```python
from build123d import *

# Parameters (mm, degrees)
SKETCH155_R     = 1.55
SKETCH155_R_2   = 2.05
SKETCH155_R_3   = 1.05
PAD061_DEPTH    = 4
POCKET077_DEPTH = 4.001
POCKET078_DEPTH = 4.001
FILLET005_R     = 0.8


with BuildPart() as part:
    # Sketch155 → Pad061 (new body)
    with BuildSketch(Plane.XY):
        with BuildLine():
            Line((-22, 28), (-45, 28))
            ThreePointArc((-45, 28), (-48.535534, 26.535534), (-50, 23))
            Line((-50, 23), (-50, 13.15))
            ThreePointArc((-51.5, 11.65), (-50.43934, 12.08934), (-50, 13.15))
            Line((-51.5, 11.65), (-54.8, 11.65))
            ThreePointArc((-54.8, 11.65), (-55.86066, 11.21066), (-56.3, 10.15))
            Line((-56.3, 10.15), (-56.3, -14.47))
            ThreePointArc((-56.3, -14.47), (-55.86066, -15.53066), (-54.8, -15.97))
            Line((-51.5, -15.97), (-54.8, -15.97))
            ThreePointArc((-50, -17.47), (-50.43934, -16.40934), (-51.5, -15.97))
            Line((-50, -17.47), (-50, -30))
            ThreePointArc((-50, -30), (-48.535534, -33.535534), (-45, -35))
            Line((-45, -35), (-22, -35))
            ThreePointArc((-22, -35), (-18.751973, -34.644122), (-15.658065, -33.593376))
            Line((-15.658065, -33.593376), (2.229785, -25.247871))
            ThreePointArc((2.229785, -25.247871), (3.702054, -23.956343), (4.25, -22.076084))
            Line((4.25, 22.076084), (4.25, -22.076084))
            ThreePointArc((4.25, 22.076084), (3.365413, 24.401942), (1.158791, 25.552129))
            Line((-17.328103, 27.72623), (1.158791, 25.552129))
            ThreePointArc((-17.328103, 27.72623), (-19.660044, 27.931499), (-22, 28))
        make_face()
        with Locations((-3, 21.75)):
            Circle(SKETCH155_R, mode=Mode.SUBTRACT)
        with Locations((-3, -21.75)):
            Circle(SKETCH155_R, mode=Mode.SUBTRACT)
        with Locations((-3, 0)):
            Circle(SKETCH155_R_2, mode=Mode.SUBTRACT)
        with Locations((-42.5, -30.7)):
            Circle(SKETCH155_R_2, mode=Mode.SUBTRACT)
        with Locations((-27.5, -30.7)):
            Circle(SKETCH155_R_2, mode=Mode.SUBTRACT)
        with Locations((-42.5, 23.3)):
            Circle(SKETCH155_R_2, mode=Mode.SUBTRACT)
        with Locations((-27.5, 23.3)):
            Circle(SKETCH155_R_2, mode=Mode.SUBTRACT)
        with Locations((-52.65, 8)):
            Circle(SKETCH155_R_3, mode=Mode.SUBTRACT)
        with Locations((-52.65, -12.32)):
            Circle(SKETCH155_R_3, mode=Mode.SUBTRACT)
    extrude(amount=PAD061_DEPTH)

    # Sketch156 (on Face31 of Pad061) → Pocket077 (cut, through all)
    with BuildSketch(Plane.XY.offset(4)):
        with BuildLine():
            Line((-42.5, -26.5), (-30.5, -26.5))
            ThreePointArc((-30.5, -26.5), (-29.085786, -25.914214), (-28.5, -24.5))
            Line((-28.5, -24.5), (-28.5, -15))
            ThreePointArc((-28.5, -15), (-29.085786, -13.585786), (-30.5, -13))
            Line((-30.5, -13), (-42.5, -13))
            ThreePointArc((-42.5, -13), (-43.914214, -13.585786), (-44.5, -15))
            Line((-44.5, -15), (-44.5, -24.5))
            ThreePointArc((-44.5, -24.5), (-43.914214, -25.914214), (-42.5, -26.5))
        make_face()
        with BuildLine():
            Line((-41, -7.5), (-32, -7.5))
            ThreePointArc((-32, -7.5), (-29.87868, -6.62132), (-29, -4.5))
            Line((-29, -4.5), (-29, 4.5))
            ThreePointArc((-29, 4.5), (-29.87868, 6.62132), (-32, 7.5))
            Line((-32, 7.5), (-41, 7.5))
            ThreePointArc((-41, 7.5), (-43.12132, 6.62132), (-44, 4.5))
            Line((-44, 4.5), (-44, -4.5))
            ThreePointArc((-44, -4.5), (-43.12132, -6.62132), (-41, -7.5))
        make_face()
        with BuildLine():
            Line((-40.5, 13), (-32.5, 13))
            ThreePointArc((-32.5, 13), (-31.085786, 13.585786), (-30.5, 15))
            Line((-30.5, 15), (-30.5, 18.5))
            ThreePointArc((-30.5, 18.5), (-31.085786, 19.914214), (-32.5, 20.5))
            Line((-32.5, 20.5), (-40.5, 20.5))
            ThreePointArc((-40.5, 20.5), (-41.914214, 19.914214), (-42.5, 18.5))
            Line((-42.5, 18.5), (-42.5, 15))
            ThreePointArc((-42.5, 15), (-41.914214, 13.585786), (-40.5, 13))
        make_face()
    extrude(amount=-POCKET077_DEPTH, mode=Mode.SUBTRACT)

    # Sketch157 (on Face5 of Pocket077) → Pocket078 (cut, through all)
    with BuildSketch(Plane.XY.offset(4)):
        with BuildLine():
            ThreePointArc((-7.582576, -2), (-4.119662, -4.873023), (0.25, -3.799671))
            Line((0.25, -3.799671), (0.25, -19.418155))
            ThreePointArc((0.25, -19.418155), (-1.755149, -17.948639), (-4.241129, -17.947422))
            Line((-4.241129, -17.947422), (-22, -2))
            Line((-22, -2), (-7.582576, -2))
        make_face()
        with BuildLine():
            ThreePointArc((-6.93352, 22.476238), (-6.999674, 21.698928), (-6.913694, 20.92356))
            Line((-22, 7.376095), (-6.913694, 20.92356))
            Line((-22, 24), (-22, 7.376095))
            ThreePointArc((-17.795293, 23.753607), (-19.89404, 23.938349), (-22, 24))
            Line((-6.93352, 22.476238), (-17.795293, 23.753607))
        make_face()
        with BuildLine():
            Line((0.25, 19.418155), (0.25, 3.799671))
            ThreePointArc((0.25, 3.799671), (-4.119662, 4.873023), (-7.582576, 2))
            Line((-22, 2), (-7.582576, 2))
            Line((-4.241129, 17.947422), (-22, 2))
            ThreePointArc((-4.241129, 17.947422), (-1.755149, 17.948639), (0.25, 19.418155))
        make_face()
        with BuildLine():
            Line((-17.349248, -29.968476), (-5.818135, -24.588681))
            ThreePointArc((-6.913694, -20.92356), (-6.832448, -22.895575), (-5.818135, -24.588681))
            Line((-6.913694, -20.92356), (-22, -7.376095))
            Line((-22, -7.376095), (-22, -31))
            ThreePointArc((-22, -31), (-19.618113, -30.739023), (-17.349248, -29.968476))
        make_face()
    extrude(amount=-POCKET078_DEPTH, mode=Mode.SUBTRACT)

    # Fillet005
    fillet005_edges = [part.edges().sort_by_distance(p)[0] for p in [
        (-22, -7.376095, 2),
        (-22, -2, 2),
        (-6.913694, -20.92356, 2),
        (-5.818135, -24.588681, 2),
        (-22, -31, 2),
        (-22, 2, 2),
        (-4.241129, 17.947422, 2),
        (0.25, 19.418155, 2),
        (-7.582576, 2, 2),
        (0.25, 3.799671, 2),
        (-22, 7.376095, 2),
        (-22, 24, 2),
        (-6.93352, 22.476238, 2),
        (-6.913694, 20.92356, 2),
        (0.25, -3.799671, 2),
        (-7.582576, -2, 2),
        (-4.241129, -17.947422, 2),
        (0.25, -19.418155, 2),
    ]]
    fillet(fillet005_edges, radius=FILLET005_R)


with BuildPart() as part_1:
    # Body023 placement: moved
    add(part.part.moved(Location((0, 0, 8.1))))


solid = part_1.part
```
Model file for the job. Use its own axes, mm. A direction names the side the tool comes from. Round coordinates to 2 decimals unless told otherwise and drop trailing zeros. Loops run counter-clockwise (first coordinate to the right, second up) from the corner with the lowest first, then second, coordinate; pieces in that order, holes last. Notation, with made-up numbers: M 47.5,-11.5 L 80.5,-11.5 A20 cw 80.5,-3.5 Z; hole C -24,13.25 d2. An arc over 180 degrees is marked long. Put each result on its own line as item: value. Start each with the question number.
Item 1: Cut at B-B (y = -6.5). List the corners of the cut face in (x, z), then the cut area to 3 significant figures.
Item 2: Drill centre lines: line 1 along Y through (x, z) = (-27.5, 9.75); line 2 along Y through (x, z) = (-52.65, 10.7); line 3 along Y through (x, z) = (-41, 8.7). Where is each one in solid material? Low to high.
Item 3: 3-axis set-ups, long thin cutter, end or side, ignore diameter. For faces 1 (the face through (-50, 18, 10)), 2 (the face through (-31.07, 19.9, 10.13)), 3 (the face through (-56.3, -2, 10)): which of +Z, -Z, +X, -X, +Y, -Y reach the whole face in a straight line?
Item 4: Cut at C-C (x = -3). List the corners of the cut face in (y, z), then the cut area to 3 significant figures.
Item 5: Mould opens along X. For faces 4 (the face through (-48, 27, 10)), 5 (the face through (-43.9, -13.57, 10.13)), 6 (the face through (-2.38, 17.8, 10.13)), 7 (the face through (-53, 11.65, 10)) say: released by +X, released by -X, zero draft, split by the parting line, or undercut.
Item 6: Cut at D-D (x = -12). List the corners of the cut face in (y, z), then the cut area to 3 significant figures.
Item 7: Drop flat-ended pins along their axis: P1, Ø1.5, axis at y = -24.5, z = 10.5, coming from the -X side; P2, Ø1.2, axis at y = 12, z = 10.5, coming from the -X side; P3, Ø1, axis at x = -53.5, z = 10.5, coming from the +Y side. Give the stop position or say it passes through.
Item 8: Cut at A-A (x = -52.65). List the corners of the cut face in (y, z).
Answer block:
1. outline: M -56.3,8.1 L -43.24,8.1 L -43.24,12.1 L -56.3,12.1 Z; M -29.76,8.1 L -16.99,8.1 L -16.99,12.1 L -29.76,12.1 Z; M 0.25,8.1 L 4.25,8.1 L 4.25,12.1 L 0.25,12.1 Z
1. area: 119 mm2
2. line 1: -35 to -32.75, -28.65 to 21.25, 25.35 to 28
2. line 2: -15.97 to -13.37, -11.27 to 6.95, 9.05 to 11.65
2. line 3: -35 to -32.1, -29.3 to -26.5, -13 to -7.5, 7.5 to 13.06, 20.44 to 21.9, 24.7 to 28
3. face 1: +Z, -Z, -X, +Y
3. face 2: +Z, -Z
3. face 3: +Z, -Z, -X, +Y, -Y
4. outline: M -27.69,8.1 L -23.3,8.1 L -23.3,12.1 L -27.69,12.1 Z; M -20.2,8.1 L -17.75,8.1 L -17.75,12.1 L -20.2,12.1 Z; M -5,8.1 L -2.05,8.1 L -2.05,12.1 L -5,12.1 Z; M 2.05,8.1 L 5,8.1 L 5,12.1 L 2.05,12.1 Z; M 17.75,8.1 L 20.2,8.1 L 20.2,12.1 L 17.75,12.1 Z; M 23.3,8.1 L 26.04,8.1 L 26.04,12.1 L 23.3,12.1 Z
4. area: 71.7 mm2
5. face 4: released by -X
5. face 5: undercut
5. face 6: undercut
5. face 7: zero draft
6. outline: M -31.89,8.1 L -27.47,8.1 L -27.47,12.1 L -31.89,12.1 Z; M -16.36,8.1 L -10.98,8.1 L -10.98,12.1 L -16.36,12.1 Z; M -2,8.1 L 2,8.1 L 2,12.1 L -2,12.1 Z; M 10.98,8.1 L 16.36,8.1 L 16.36,12.1 L 10.98,12.1 Z; M 23.07,8.1 L 27.1,8.1 L 27.1,12.1 L 23.07,12.1 Z
6. area: 92.8 mm2
7. P1: x = -50
7. P2: x = -55.63
7. P3: y = 11.65
8. outline: M -15.97,8.1 L -13.37,8.1 L -13.37,12.1 L -15.97,12.1 Z; M -11.27,8.1 L 6.95,8.1 L 6.95,12.1 L -11.27,12.1 Z; M 9.05,8.1 L 11.65,8.1 L 11.65,12.1 L 9.05,12.1 Z
